Here's the drawing with two shaded views (mm, measured from the low corner). I have some questions. A direction names the side the tool comes from. Round coordinates to 2 decimals unless told otherwise and drop trailing zeros. Order: outer loops, then holes, each group sorted by start corner. A loop starts at its lowest first (then second) coordinate and runs counter-clockwise, first axis right, second up. Notation, with made-up numbers: (52, 35) -> (97, 35) arc R9 ccw to (97, 44) -> close; hole circle Ø1 at (33.5, -12). An arc over 180 degrees is marked (long way). Use a Markdown table: item, result. Add a question column.
Q1. I'm going to push flat-ended pins straight in: pin 1 Ø6 at (x, z) = (6, 41) entering from +Y; pin 2 Ø10 at (y, z) = (9, 7.5) entering from -X; pin 3 Ø3 at (y, z) = (44.5, 45) entering from +X; pin 4 Ø7 at (y, z) = (45, 5) entering from +X. Where does each tip first touch, or does it pass through?
Q2. For the marked faces 1 and 2, which set-ups out of +Z, -Z, +X, -X, +Y, -Y let a thin tool reach every point of the face, with its end or its side?
Q3. If we section it at B-B on y = 45: List the corners of the cut face in (x, z) for me, plus the area to 3 significant figures.
Q4. If we section it at D-D on x = 3.5: List the corners of the cut face in (y, z) for me, plus the area to 3 significant figures.
Q5. If we section it at C-C on y = 5: List the corners of the cut face in (x, z) for me, plus the area to 3 significant figures.
Q6. If we section it at A-A on z = 5: List the corners of the cut face in (x, y) for me.
Q7. I need wall thicknesses on line 1 along Y through (x, z) = (0.6, 5); line 2 along X through (y, z) = (38, 7.5); line 3 along Z through (x, y) = (17.5, 3.5). Which ranges of each line are inside material? Lowest first, please. Write a range as [from, to].
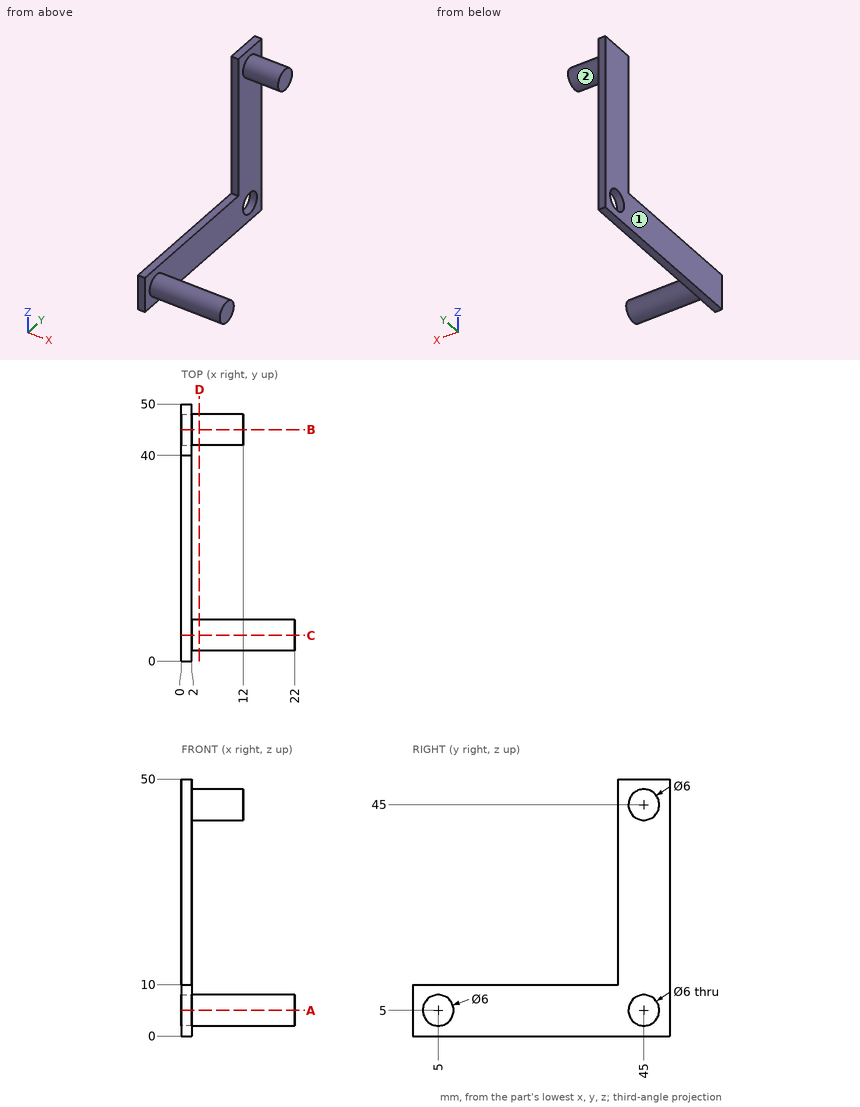
Answer below:
| question | item | result |
|---|---|---|
| 1 | pin 1 | y = 47.83 |
| 1 | pin 2 | x = 0 |
| 1 | pin 3 | x = 12 |
| 1 | pin 4 | x = 2 |
| 2 | face 1 | +Z, -Z, -X, +Y, -Y |
| 2 | face 2 | +X |
| 3 | outline | (0, 0) -> (2, 0) -> (2, 2) -> (0, 2) -> close; (0, 8) -> (2, 8) -> (2, 42) -> (12, 42) -> (12, 48) -> (2, 48) -> (2, 50) -> (0, 50) -> close |
| 3 | area | 148 mm² |
| 4 | outline | circle Ø6 at (5, 5); circle Ø6 at (45, 45) |
| 4 | area | 56.5 mm² |
| 5 | outline | (0, 0) -> (2, 0) -> (2, 2) -> (22, 2) -> (22, 8) -> (2, 8) -> (2, 10) -> (0, 10) -> close |
| 5 | area | 140 mm² |
| 6 | outline | (0, 0) -> (2, 0) -> (2, 2) -> (22, 2) -> (22, 8) -> (2, 8) -> (2, 42) -> (0, 42) -> close; (0, 48) -> (2, 48) -> (2, 50) -> (0, 50) -> close |
| 7 | line 1 | [0, 42], [48, 50] |
| 7 | line 2 | [0, 2] |
| 7 | line 3 | [2.4, 7.6] |
